from build123d import *

# Parameters (mm, degrees)
SKETCH2_R          = 1.25
CUT_EXTRUDE1_DEPTH = 10
SKETCH4_R          = 1.25
CUT_EXTRUDE2_DEPTH = 10


with BuildPart() as part:
    # Sketch1 → Revolve1 (revolve)
    with BuildSketch(Plane.XY):
        Polygon((7.5, 57.821876273), (7.5, 7.221876273), (15, 7.221876273), (15, 13.686423943), (25, 13.686423943), (25, 17.186423943), (21, 17.186423943), (21, 55.321876273), (17.801767056, 55.321876273), (17.801767056, 57.821876273), align=None)
        Polygon((8.7, 53.521876273), (19.6, 53.521876273), (19.6, 15.931935651), (13.113770226, 15.931935651), (13.113770226, 12.516887812), (8.7, 12.516887812), align=None, mode=Mode.SUBTRACT)
    revolve(axis=Axis((0, 0, 0), (0, 1, 0)))

    # Sketch2 → Cut-Extrude1 (cut)
    with BuildSketch(Plane(origin=(0, 17.186423943, 0), x_dir=(1, 0, 0), z_dir=(0, 1, 0))):
        with Locations((0, 23)):
            Circle(SKETCH2_R)
        with Locations((19.918584287, 11.5)):
            Circle(SKETCH2_R)
        with Locations((19.918584287, -11.5)):
            Circle(SKETCH2_R)
        with Locations((0, -23)):
            Circle(SKETCH2_R)
        with Locations((-19.918584287, -11.5)):
            Circle(SKETCH2_R)
        with Locations((-19.918584287, 11.5)):
            Circle(SKETCH2_R)
    extrude(amount=-CUT_EXTRUDE1_DEPTH, mode=Mode.SUBTRACT)

    # Sketch4 → Cut-Extrude2 (cut)
    with BuildSketch(Plane(origin=(0, 12.516887812, 0), x_dir=(1, 0, 0), z_dir=(0, 1, 0))):
        with Locations((0, 11)):
            Circle(SKETCH4_R)
        with Locations((9.526279442, 5.5)):
            Circle(SKETCH4_R)
        with Locations((9.526279442, -5.5)):
            Circle(SKETCH4_R)
        with Locations((0, -11)):
            Circle(SKETCH4_R)
        with Locations((-9.526279442, -5.5)):
            Circle(SKETCH4_R)
        with Locations((-9.526279442, 5.5)):
            Circle(SKETCH4_R)
    extrude(amount=-CUT_EXTRUDE2_DEPTH, mode=Mode.SUBTRACT)


solid = part.part
Part model, mm, in its own coordinate system. A direction names the side the tool comes from. Give positions to 0.01 mm unless a question says otherwise; leave off trailing zeros. Order: outer loops, then holes, each group sorted by start corner. A loop starts at its lowest first (then second) coordinate and runs counter-clockwise, first axis right, second up. Notation, with made-up numbers: (-27.5, 49.25) - (-5.5, 49.25) arc R31 cw to (-5.5, 80.25) - close; hole circle Ø8 at (19, 34.25). An arc over 180 degrees is marked (long way). One line per question, with ' | ' between items.
1. Drill centre lines: probe 1 along Z at (x, y) = (0.5, 41.5); probe 2 along Z at (x, y) = (-20, 16.5); probe 3 along Z at (x, y) = (0, 8.5). Where is each one in solid material? Low to high.
Filled in:
probe 1: -20.99 to -19.59, -8.69 to -7.48, 7.48 to 8.69, 19.59 to 20.99 | probe 2: -15 to -12.75, -10.25 to 10.25, 12.75 to 15 | probe 3: -15 to -12.25, -9.75 to -7.5, 7.5 to 9.75, 12.25 to 15
2. Band-saw the part on B-B on z = 2.5. Give the number of separate pieces and of enclosed holes in the cut face, then the cut area to 3 significant figures.
Filled in:
separate pieces: 2 | enclosed holes: 2 | area: 462 mm²
3. Band-saw the part on A-A on y = 30.5. List the corners of the cut face in (x, z), then the cut area to 3 significant figures.
Filled in:
outline: circle Ø42 at (0, 0); circle Ø17.4 at (0, 0); hole circle Ø39.2 at (0, 0); hole circle Ø15 at (0, 0) | area: 240 mm²
4. Band-saw the part on D-D on z = 23. List the corners of the cut face in (x, y).
Filled in:
outline: (-9.8, 13.69) - (-1.25, 13.69) - (-1.25, 17.19) - (-9.8, 17.19) - close; (1.25, 13.69) - (9.8, 13.69) - (9.8, 17.19) - (1.25, 17.19) - close
5. Pull direction X, two halves, no side cores. Call faces 4 (the face through (-5.7, 17.186, -20.5)), 5 (the face through (-4.249, 34.464, 19.134)), 6 (the face through (23.846, 15.461, -7.509)): +X half, -X half, draft (parallel to the pull), parting line (faces both ways), or undercut.
Filled in:
face 4: draft | face 5: undercut | face 6: parting line
6. Drop flat-ended pins along their axis: P1, Ø3, axis at x = 14, z = -14, coming from the +Y side; P2, Ø3, axis at x = 19.92, z = -11.5, coming from the +Y side; P3, Ø3, axis at x = 9.5, z = 15, coming from the -Y side; P4, Ø19.5, axis at x = 1.5, z = -3.5, coming from the +Y side. Give the stop position or say it passes through.
Filled in:
P1: y = 55.32 | P2: y = 17.19 | P3: y = 13.69 | P4: y = 57.82
7. Which spindle directions (+Z, -Z, +X, -X, +Y, -Y) get a long thin tool onto all of the face, cutting with end or side? Do faces 1 (the face through (-3.86, 56.59, 17.38)), 2 (the face through (-0.16, 9.91, 9.76)), 3 (the face through (-1.886, 33.306, 8.493)). Say none if no direction does.
Filled in:
face 1: +Y | face 2: -Y | face 3: none
